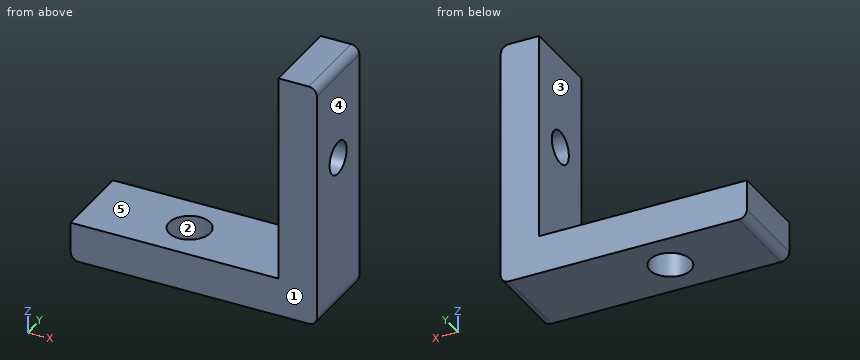
```python
from build123d import *

# Parameters (mm, degrees)
F0_W     = 25.4
F0_H     = 10
F0_R     = 2.5
F1_DEPTH = 4.7
F2_W     = 10
F2_H     = 30.1
F2_R     = 2
F3_DEPTH = 4.7
F4_R     = 1


with BuildPart() as f1:
    # F0 (on Top) → F1 (new body)
    with BuildSketch(Plane.XY):
        Rectangle(F0_W, F0_H)
        with Locations((-0.75, 0)):
            Circle(F0_R, mode=Mode.SUBTRACT)
    extrude(amount=F1_DEPTH)

    # F2 (on face) → F3 (join)
    with BuildSketch(Plane.YZ.offset(12.7)):
        with Locations((0, 15.05)):
            Rectangle(F2_W, F2_H)
        with Locations((0, 18.65)):
            Circle(F2_R, mode=Mode.SUBTRACT)
    extrude(amount=F3_DEPTH)

    # F4
    f4_edges = [f1.edges().sort_by_distance(p)[0] for p in [
        (17.4, 0, 30.1),
        (17.4, 0, 0),
        (-12.7, 0, 0),
    ]]
    fillet(f4_edges, radius=F4_R)


solid = f1.part
```
Input: part model. Units: mm. Frame: model coordinates. Face numbers are marked on the shaded views. A direction names the side the tool comes from. Give positions to 0.01 mm unless a question says otherwise; leave off trailing zeros. Loops run counter-clockwise (first coordinate to the right, second up) from the corner with the lowest first, then second, coordinate; pieces in that order, holes last. Notation, with made-up numbers: (25, 76.25) -> (63, 76.25) arc R12 cw to (63, 96.25) -> close; hole circle Ø6 at (25, -23.5). An arc over 180 degrees is marked (long way). Use a Markdown table: item, result.
Q1. Section query C-C, the plane z = 18.65. Return the cut outline in (x, y), plus the area to 3 significant figures.
Entries:
| item | result |
|---|---|
| outline | (12.7, -5) -> (17.4, -5) -> (17.4, -2) -> (12.7, -2) -> close; (12.7, 2) -> (17.4, 2) -> (17.4, 5) -> (12.7, 5) -> close |
| area | 28.2 mm² |
Q2. Access query for the marked faces 4 and 5. Directions: +Z, -Z, +X, -X, +Y, -Y. A direction counts if a zero-diameter tool reaches every point of the face in a straight line with its end or side. Return the directions, or none.
Entries:
| item | result |
|---|---|
| face 4 | +Z, -Z, +X, +Y, -Y |
| face 5 | +Z, -X, +Y, -Y |
Q3. First-contact query: P1, Ø4, axis at x = 9, y = -1.5, coming from the +Z side; P2, Ø5, axis at y = 0.5, z = 16, coming from the -X side. Flat tips, straight axial feed; report the tip coordinate or a pass-through.
Entries:
| item | result |
|---|---|
| P1 | stops at z = 4.7 |
| P2 | stops at x = 12.7 |
Q4. Pull-direction query (X, two-part tool) for the marked faces 1, 2 and 3; classes: pulls with the +X half, pulls with the -X half, needs draft (parallel to the pull), parting line crosses it, or undercut.
Entries:
| item | result |
|---|---|
| face 1 | needs draft |
| face 2 | undercut |
| face 3 | pulls with the -X half |
Q5. Section query D-D, the plane y = -3.75. Return the cut outline in (x, z).
Entries:
| item | result |
|---|---|
| outline | (-12.7, 1) arc R1 ccw to (-11.7, 0) -> (16.4, 0) arc R1 ccw to (17.4, 1) -> (17.4, 29.1) arc R1 ccw to (16.4, 30.1) -> (12.7, 30.1) -> (12.7, 4.7) -> (-12.7, 4.7) -> close |
Q6. Section query A-A, the plane y = 0. Return the cut outline in (x, z), plus the area to 3 significant figures.
Entries:
| item | result |
|---|---|
| outline | (-12.7, 1) arc R1 ccw to (-11.7, 0) -> (-3.25, 0) -> (-3.25, 4.7) -> (-12.7, 4.7) -> close; (1.75, 0) -> (16.4, 0) arc R1 ccw to (17.4, 1) -> (17.4, 16.65) -> (12.7, 16.65) -> (12.7, 4.7) -> (1.75, 4.7) -> close; (12.7, 20.65) -> (17.4, 20.65) -> (17.4, 29.1) arc R1 ccw to (16.4, 30.1) -> (12.7, 30.1) -> close |
| area | 218 mm² |
Q7. Section query B-B, the plane x = -0.75. Return the cut outline in (y, z), plus the area to 3 significant figures.
Entries:
| item | result |
|---|---|
| outline | (-5, 0) -> (-2.5, 0) -> (-2.5, 4.7) -> (-5, 4.7) -> close; (2.5, 0) -> (5, 0) -> (5, 4.7) -> (2.5, 4.7) -> close |
| area | 23.5 mm² |
Q8. Ray query, probe 1 along Y at (x, z) = (-0.75, 1.8); probe 2 along Z at (x, y) = (8, -2.5); probe 3 along X at (y, z) = (4.5, 28.5). Return the intervals inside material, ascending. Write a range as from..to.
Entries:
| item | result |
|---|---|
| probe 1 | y = -5..-2.5, 2.5..5 |
| probe 2 | z = 0..4.7 |
| probe 3 | x = 12.7..17.4 |
